Job drawing, mm, ordinate dimensions from the low corner. One solid piece. A direction names the side the tool comes from. Round coordinates to 2 decimals unless told otherwise and drop trailing zeros. Write each loop counter-clockwise with the first axis right and the second up, starting at its lowest first coordinate (ties: lowest second). Pieces come first, ordered by that corner, then holes.
1) Saw through at B-B (y = 14.5). Write the cut outline in (x, z).
2) Pull direction Y, two halves, no side cores. Call the marked faces 3, 4, 5 and 6: +Y half, -Y half, draft (parallel to the pull), parting line (faces both ways), or undercut.
3) Saw through at C-C (x = 5.75). Write the cut outline in (y, z).
4) Which spindle directions (+Z, -Z, +X, -X, +Y, -Y) get a long thin tool onto all of the face, cutting with end or side? Do the marked faces 1 and 2. Say none if no direction does.
5) Wall check: probe 1 along X at (y, z) = (10.75, 0.9); probe 2 along Y at (x, z) = (6, 2.05); probe 3 along X at (y, z) = (2.25, 2.4) (1 decimal). Give the ranges that are in metal, low to high.
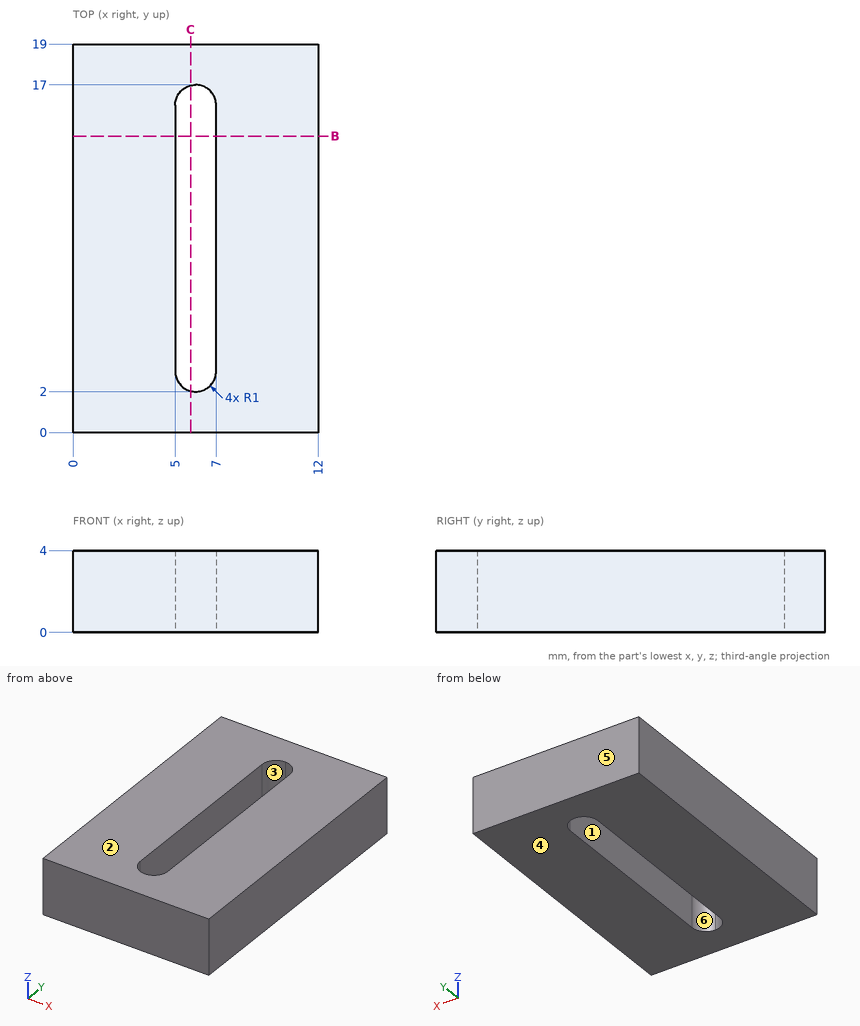
Evaluation:
1. outline: (0, 0) - (5, 0) - (5, 4) - (0, 4) - close; (7, 0) - (12, 0) - (12, 4) - (7, 4) - close
2. face 3: undercut
2. face 4: draft
2. face 5: +Y half
2. face 6: undercut
3. outline: (0, 0) - (2.03, 0) - (2.03, 4) - (0, 4) - close; (16.97, 0) - (19, 0) - (19, 4) - (16.97, 4) - close
4. face 1: +Z, -Z
4. face 2: +Z, +X, -X, +Y, -Y
5. probe 1: x = 0 to 5, 7 to 12
5. probe 2: y = 0 to 2, 17 to 19
5. probe 3: x = 0 to 5.3, 6.7 to 12
